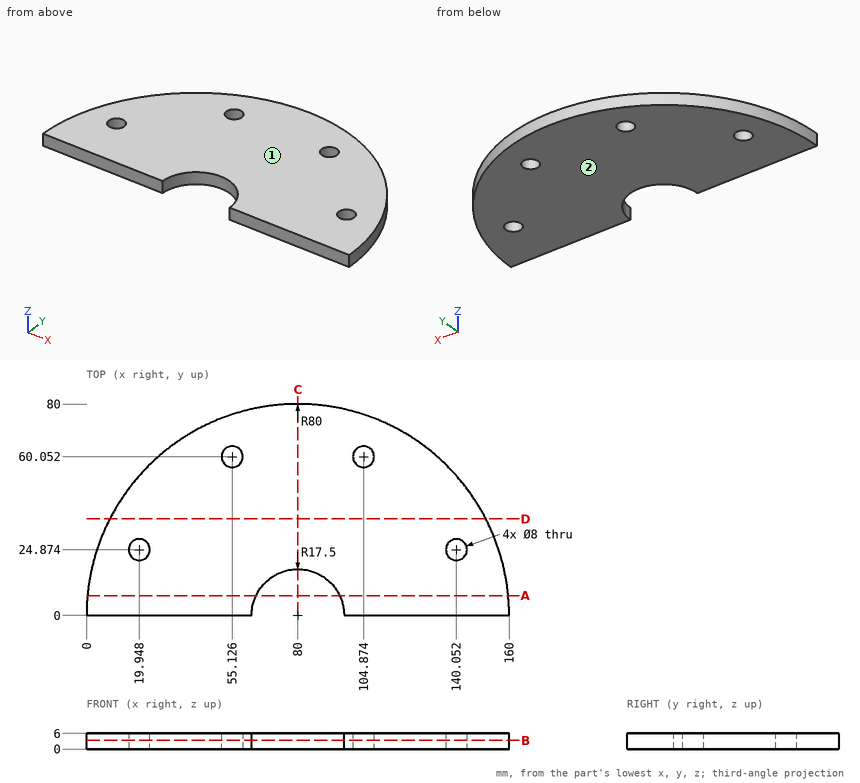
Input: dimensioned drawing with shaded views. Units: mm. Origin: part minimum x, y, z. Round coordinates to 2 decimals unless told otherwise and drop trailing zeros. Loops run counter-clockwise (first coordinate to the right, second up) from the corner with the lowest first, then second, coordinate; pieces in that order, holes last. Notation, with made-up numbers: (16, 19) -> (65, 19) arc R10 cw to (65, 33) -> close; hole circle Ø9 at (81.5, 76.25). An arc over 180 degrees is marked (long way). One line per item, written item: value.
(1) Section C-C (x = 80). Return the cut outline in (y, z).
Geometry check:
outline: (17.5, 0) -> (80, 0) -> (80, 6) -> (17.5, 6) -> close
(2) Mould query, pull axis Z, two halves, no side actions, for the marked faces 1 and 2. Classes: pulls with the +Z half, pulls with the -Z half, needs draft (parallel to the pull), parting line crosses it, or undercut.
Geometry check:
face 1: pulls with the +Z half
face 2: pulls with the -Z half
(3) Section B-B (z = 3.3). Return the cut outline in (x, y) (1 decimal).
Geometry check:
outline: (0, 0) -> (62.5, 0) arc R17.5 cw to (97.5, 0) -> (160, 0) arc R80 ccw to start; hole circle Ø8 at (19.9, 24.9); hole circle Ø8 at (55.1, 60.1); hole circle Ø8 at (104.9, 60.1); hole circle Ø8 at (140.1, 24.9)
(4) Section A-A (y = 7.5). Return the cut outline in (x, z), plus the area to 3 significant figures.
Geometry check:
outline: (0.35, 0) -> (64.19, 0) -> (64.19, 6) -> (0.35, 6) -> close; (95.81, 0) -> (159.65, 0) -> (159.65, 6) -> (95.81, 6) -> close
area: 766 mm2
(5) Material intervals for line 1 (X direction, y = 56.5, z = 4) (1 decimal); line 2 (X direction, y = 21.5, z = 2.3) (1 decimal); line 3 (X direction, y = 11, z = 1.4), sorted ascending. Write a range as [from, to].
Geometry check:
line 1: [23.4, 53.3], [57, 103], [106.7, 136.6]
line 2: [2.9, 17.8], [22.1, 137.9], [142.2, 157.1]
line 3: [0.76, 66.39], [93.61, 159.24]
(6) Pin query (flat end, axial travel): pin 1 (1.5 mm diameter, centred on y = 16.5, z = 2, fed in from -X); pin 2 (3 mm diameter, centred on y = 34, z = 2, fed in from -X); pin 3 (2 mm diameter, centred on x = 91, z = 2, fed in from +Y). Return the tip coordinate at first contact, or that it passes through.
Geometry check:
pin 1: x = 1.57
pin 2: x = 6.9
pin 3: y = 79.37
(7) Section D-D (y = 36.5). Return the cut outline in (x, z).
Geometry check:
outline: (8.81, 0) -> (151.19, 0) -> (151.19, 6) -> (8.81, 6) -> close
